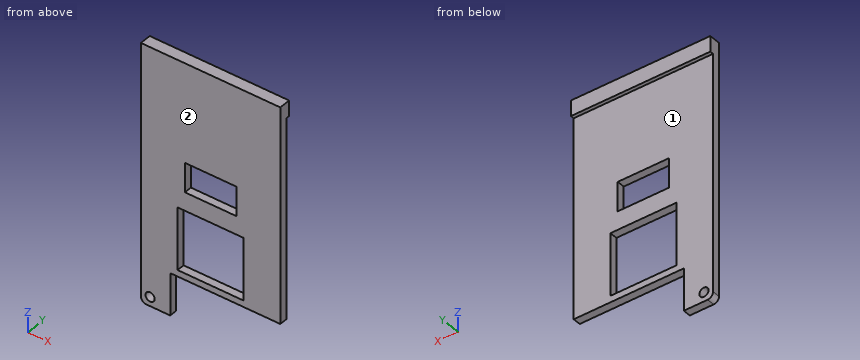
from build123d import *

# Parameters (mm, degrees)
BOSS_EXTRUDE1_OUTLINE_W   = 14
BOSS_EXTRUDE1_OUTLINE_H   = 8
BOSS_EXTRUDE1_OUTLINE_R   = 1.25
BOSS_EXTRUDE1_OUTLINE_W_2 = 18
BOSS_EXTRUDE1_OUTLINE_H_2 = 17
BOSS_EXTRUDE1_DEPTH       = 2.13
SKETCH2_W                 = 38
SKETCH2_H                 = 4.23
BOSS_EXTRUDE2_DEPTH       = 1
SKETCH3_W                 = 8
SKETCH3_H                 = 2.13
CUT_EXTRUDE1_DEPTH        = 11.5


# Read off the part's stored shape, not the designer's step: Boss-Extrude1
with BuildPart() as part:
    # Boss-Extrude1 outline → Boss-Extrude1 (new body)
    with BuildSketch(Plane(origin=(0, 0, 0), x_dir=(1, 0, 0), z_dir=(0, 1, 0))):
        with BuildLine():
            ThreePointArc((38, 88), (37.560660172, 89.060660172), (36.5, 89.5))
            Line((36.5, 89.5), (30, 89.5))
            Line((30, 89.5), (30, 78))
            Line((30, 78), (8, 78))
            Line((8, 78), (8, 89.5))
            Line((8, 89.5), (1.5, 89.5))
            ThreePointArc((1.5, 89.5), (0.439339828, 89.060660172), (0, 88))
            Line((0, 88), (0, 19.25))
            Line((0, 19.25), (38, 19.25))
            Line((38, 19.25), (38, 88))
        make_face()
        with Locations((19, 50.25)):
            Rectangle(BOSS_EXTRUDE1_OUTLINE_W, BOSS_EXTRUDE1_OUTLINE_H, mode=Mode.SUBTRACT)
        with Locations((2.5, 87)):
            Circle(BOSS_EXTRUDE1_OUTLINE_R, mode=Mode.SUBTRACT)
        with Locations((19, 67.75)):
            Rectangle(BOSS_EXTRUDE1_OUTLINE_W_2, BOSS_EXTRUDE1_OUTLINE_H_2, mode=Mode.SUBTRACT)
        with Locations((35.5, 87)):
            Circle(BOSS_EXTRUDE1_OUTLINE_R, mode=Mode.SUBTRACT)
    extrude(amount=BOSS_EXTRUDE1_DEPTH)

    # Sketch2 → Boss-Extrude2 (add)
    with BuildSketch(Plane(origin=(0, 2.13, 0), x_dir=(1, 0, 0), z_dir=(0, 1, 0))):
        with Locations((19, 21.365)):
            Rectangle(SKETCH2_W, SKETCH2_H)
    extrude(amount=BOSS_EXTRUDE2_DEPTH)

    # Sketch3 → Cut-Extrude1 (cut)
    with BuildSketch(Plane(origin=(0, 0, -89.5), x_dir=(-1, 0, 0), z_dir=(0, 0, -1))):
        with Locations((-34, 1.065)):
            Rectangle(SKETCH3_W, SKETCH3_H)
    extrude(amount=-CUT_EXTRUDE1_DEPTH, mode=Mode.SUBTRACT)


solid = part.part
Work out the finished part from the listing and answer in its coordinate system (mm). Face numbers are marked on the shaded views. A direction names the side the tool comes from. Round coordinates to 2 decimals unless told otherwise and drop trailing zeros. Loops run counter-clockwise (first coordinate to the right, second up) from the corner with the lowest first, then second, coordinate; pieces in that order, holes last. Notation, with made-up numbers: M 19.5,27 L 58.5,27 A33 cw 58.5,59 Z; hole C 70,75 d10. An arc over 180 degrees is marked long. One line per question, with ' | ' between items. Start each with the question number.
(1) A cutting plane is placed at B-B on y = 1.3. Write down the section's boundary in (x, z).
(2) A cutting plane is placed at D-D on z = -87. Write down the section's boundary in (x, y).
(3) A cutting plane is placed at A-A on x = 21.5. Write down the section's boundary in (y, z), plus the area to 3 significant figures.
(4) Flat-ended cylindrical pins translate along their axes: pin 1 Ø8 at (x, z) = (11, -42.5) entering from +Y; pin 2 Ø1.1 at (x, y) = (18, 1) entering from -Z; pin 3 Ø0.6 at (y, z) = (0.5, -83) entering from +X. Find the tip coordinate at first contact, or state that the pin passes through.
(5) Find the intervals of material crossed by line 1 (Z direction, x = 13, y = 1.75); line 2 (X direction, y = 1.55, z = -52); line 3 (Z direction, x = 2.5, y = 1.3), in increasing order.
(6) A tool of negligible diameter and unlimited length cuts with its end or side. For the marked faces 1 and 2, from which of +Z, -Z, +X, -X, +Y, -Y can it reach the whole face along a straight path? Write none if from no direction.
(7) A cutting plane is placed at C-C on x = 2.5. Write down the section's boundary in (y, z), plus the area to 3 significant figures.
Geometry check:
1) outline: M 0,-88 A1.5 ccw 1.5,-89.5 L 8,-89.5 L 8,-78 L 38,-78 L 38,-19.25 L 0,-19.25 Z; hole C 2.5,-87 d2.5; hole M 10,-76.25 L 28,-76.25 L 28,-59.25 L 10,-59.25 Z; hole M 12,-54.25 L 26,-54.25 L 26,-46.25 L 12,-46.25 Z
2) outline: M 0,0 L 1.25,0 L 1.25,2.13 L 0,2.13 Z; M 3.75,0 L 8,0 L 8,2.13 L 3.75,2.13 Z
3) outline: M 0,-78 L 2.13,-78 L 2.13,-76.25 L 0,-76.25 Z; M 0,-59.25 L 2.13,-59.25 L 2.13,-54.25 L 0,-54.25 Z; M 0,-46.25 L 2.13,-46.25 L 2.13,-23.48 L 3.13,-23.48 L 3.13,-19.25 L 0,-19.25 Z | area: 76.1 mm²
4) pin 1: stops at y = 2.13 | pin 2: stops at z = -78 | pin 3: stops at x = 8
5) line 1: z = -78 to -76.25, -59.25 to -54.25, -46.25 to -19.25 | line 2: x = 0 to 12, 26 to 38 | line 3: z = -89.5 to -88.25, -85.75 to -19.25
6) face 1: -Z, +X, -X, +Y | face 2: +Z, -Z, +X, -X, -Y
7) outline: M 0,-89.5 L 2.13,-89.5 L 2.13,-88.25 L 0,-88.25 Z; M 0,-85.75 L 2.13,-85.75 L 2.13,-23.48 L 3.13,-23.48 L 3.13,-19.25 L 0,-19.25 Z | area: 149 mm²
